Design review of the part built by this model. Coordinates are the model's own, in mm. A direction names the side the tool comes from. Give positions to 0.01 mm unless a question says otherwise; leave off trailing zeros. Write each loop counter-clockwise with the first axis right and the second up, starting at its lowest first coordinate (ties: lowest second). Pieces come first, ordered by that corner, then holes. Notation, with made-up numbers: (-0.75, 26) - (47.25, 26) arc R27 ccw to (47.25, 59) - close; hole circle Ø5 at (-8, 33.5). An arc over 180 degrees is marked (long way). Use a Markdown table: item, result. Add a question column.
```python
from build123d import *

# Parameters (mm, degrees)
EXTRUDE_1_DEPTH     = 20
CUT_EXTRUDE_2_DEPTH = 20


with BuildPart() as part:
    # 草图1 → 凸台-拉伸1 (new body)
    with BuildSketch(Plane(origin=(0, 0, 0), x_dir=(1, 0, 0), z_dir=(0, 1, 0))):
        Polygon((5, 2), (8, 2), (8, -2), (-8, -2), (-8, 2), (-5, 2), (-5, 4), (5, 4), align=None)
    extrude(amount=EXTRUDE_1_DEPTH)

    # 草图4 → 切除-拉伸2 (cut)
    with BuildSketch(Plane(origin=(0, 0, -4), x_dir=(-1, 0, 0), z_dir=(0, 0, -1))):
        with BuildLine():
            ThreePointArc((2, 10), (1.051462224, 11.701301617), (-0.894427191, 11.788854382))
            Line((-0.894427191, 11.788854382), (0.894427191, 8.211145618))
            ThreePointArc((0.894427191, 8.211145618), (1.701301617, 8.948537776), (2, 10))
        make_face()
        with BuildLine():
            Line((0.894427191, 8.211145618), (-0.894427191, 11.788854382))
            ThreePointArc((-0.894427191, 11.788854382), (-1.788854382, 9.105572809), (0.894427191, 8.211145618))
        make_face()
    extrude(amount=-CUT_EXTRUDE_2_DEPTH, mode=Mode.SUBTRACT)


solid = part.part
```
(1) Add section A-A (x = 0). State the section outline as (y, z) points.
(2) Insertion check: pin 1 (0.6 mm diameter, centred on y = 12.5, z = -3, fed in from -X); pin 2 (2 mm diameter, centred on y = 6.5, z = -3.5, fed in from +X); pin 3 (0.9 mm diameter, centred on x = 7, y = 14.5, fed in from -Z). Each pin has a flat end and moves straight along its axis. Give the tip position at first contact, or say it passes through.
(3) Add section B-B (y = 10.25). State the section outline as (x, z) points, and give its area (3 significant figures).
(4) Tool access review of faces 1 (the face through (-7, 10, -2)), 2 (the face through (8, 10, 0)), 3 (the face through (5, 10, -3)): name each direction out of +Z, -Z, +X, -X, +Y, -Y from which nothing blocks a thin tool from reaching the whole face with its end or side.
(5) Add section C-C (z = -0.6). State the section outline as (x, y) points, and give its area (3 significant figures).
(6) For line 1 along Z through (x, y) = (7.25, 16.75); line 2 along Y through (x, z) = (-0.75, -1.65); line 3 along X through (y, z) = (10.25, -2.9), list the stretches that pass through material, from the lowest coordinate up.
(7) Add section D-D (y = 15.75). State the section outline as (x, z) points, and give its area (3 significant figures).
Answers follow:
| question | item | result |
|---|---|---|
| 1 | outline | (0, -4) - (8, -4) - (8, 2) - (0, 2) - close; (12, -4) - (20, -4) - (20, 2) - (12, 2) - close |
| 2 | pin 1 | x = -5 |
| 2 | pin 2 | x = 5 |
| 2 | pin 3 | z = -2 |
| 3 | outline | (-8, -2) - (-5, -2) - (-5, -4) - (-1.98, -4) - (-1.98, 2) - (-8, 2) - close; (1.98, -4) - (5, -4) - (5, -2) - (8, -2) - (8, 2) - (1.98, 2) - close |
| 3 | area | 60.2 mm^2 |
| 4 | face 1 | -Z, -X, +Y, -Y |
| 4 | face 2 | +Z, -Z, +X, +Y, -Y |
| 4 | face 3 | -Z, +X, +Y, -Y |
| 5 | outline | (-8, 0) - (8, 0) - (8, 20) - (-8, 20) - close; hole circle Ø4 at (0, 10) |
| 5 | area | 307 mm^2 |
| 6 | line 1 | -2 to 2 |
| 6 | line 2 | 0 to 8.15, 11.85 to 20 |
| 6 | line 3 | -5 to -1.98, 1.98 to 5 |
| 7 | outline | (-8, -2) - (-5, -2) - (-5, -4) - (5, -4) - (5, -2) - (8, -2) - (8, 2) - (-8, 2) - close |
| 7 | area | 84.0 mm^2 |
